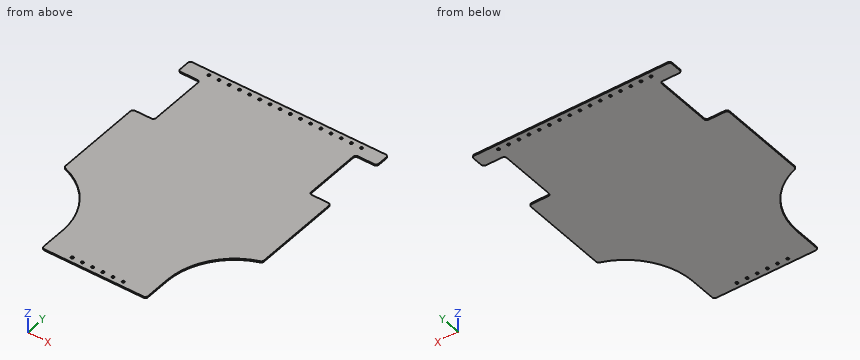
from build123d import *

# Parameters (mm, degrees)
BOSS_EXTRUDE1_DEPTH = 3.175
CUT_EXTRUDE1_DEPTH  = 403.674624387
SKETCH3_W           = 260.35
SKETCH3_H           = 3.175
BOSS_EXTRUDE2_DEPTH = 12.7
FILLET1_R           = 6.35
SKETCH5_R           = 3.175
CUT_EXTRUDE2_DEPTH  = 413.762211358


with BuildPart() as part:
    # Sketch1 → Boss-Extrude1 (new body)
    with BuildSketch(Plane.XY):
        Polygon((-247.65, 127), (-247.65, -317.5), (247.65, -317.5), (247.65, 127), (193.675, 127), (193.675, 279.4), (247.65, 279.4), (247.65, 317.5), (-247.65, 317.5), (-247.65, 279.4), (-193.675, 279.4), (-193.675, 127), align=None)
    extrude(amount=BOSS_EXTRUDE1_DEPTH)

    # Sketch2 → Cut-Extrude1 (cut, through all)
    with BuildSketch(Plane(origin=(0, 0, 0), x_dir=(-1, 0, 0), z_dir=(0, 0, -1))):
        with BuildLine():
            Line((-130.175, -260.35), (-130.175, -324.332629374))
            Line((-130.175, -324.332629374), (-142.81356865, -324.332629374))
            ThreePointArc((-142.81356865, -324.332629374), (-463.535123664, -227.740529446), (-130.175, -260.35))
        make_face()
        with BuildLine():
            Line((130.175, -324.332629374), (142.81356865, -324.332629374))
            ThreePointArc((142.81356865, -324.332629374), (463.535123664, -227.740529446), (130.175, -260.35))
            Line((130.175, -260.35), (130.175, -324.332629374))
        make_face()
    extrude(amount=-CUT_EXTRUDE1_DEPTH, mode=Mode.SUBTRACT)

    # Sketch3 → Boss-Extrude2 (add)
    with BuildSketch(Plane.XZ.offset(317.5)):
        with Locations((0, 1.5875)):
            Rectangle(SKETCH3_W, SKETCH3_H)
    extrude(amount=BOSS_EXTRUDE2_DEPTH)

    # Fillet1
    fillet1_edges = [part.edges().sort_by_distance(p)[0] for p in [
        (-247.65, 317.5, 1.5875),
        (247.65, 317.5, 1.5875),
        (247.65, 279.4, 1.5875),
        (193.675, 279.4, 1.5875),
        (193.675, 127, 1.5875),
        (247.65, 127, 1.5875),
        (-247.65, 127, 1.5875),
        (-193.675, 127, 1.5875),
        (-193.675, 279.4, 1.5875),
        (-247.65, 279.4, 1.5875),
        (247.65, -99.926075272, 1.5875),
        (-247.65, -99.926075272, 1.5875),
        (-130.175, -330.2, 1.5875),
        (130.175, -330.2, 1.5875),
    ]]
    fillet(fillet1_edges, radius=FILLET1_R)

    # Sketch5 → Cut-Extrude2 (cut, through all)
    with BuildSketch(Plane(origin=(0, 0, 0), x_dir=(-1, 0, 0), z_dir=(0, 0, -1))):
        with Locations((63.5, -317.5)):
            Circle(SKETCH5_R)
        with Locations((38.1, -317.5)):
            Circle(SKETCH5_R)
        with Locations((12.7, -317.5)):
            Circle(SKETCH5_R)
        with Locations((-12.7, -317.5)):
            Circle(SKETCH5_R)
        with Locations((-38.1, -317.5)):
            Circle(SKETCH5_R)
        with Locations((-63.5, -317.5)):
            Circle(SKETCH5_R)
        with Locations((190.5, 304.8)):
            Circle(SKETCH5_R)
        with Locations((165.1, 304.8)):
            Circle(SKETCH5_R)
        with Locations((139.7, 304.8)):
            Circle(SKETCH5_R)
        with Locations((114.3, 304.8)):
            Circle(SKETCH5_R)
        with Locations((88.9, 304.8)):
            Circle(SKETCH5_R)
        with Locations((63.5, 304.8)):
            Circle(SKETCH5_R)
        with Locations((38.1, 304.8)):
            Circle(SKETCH5_R)
        with Locations((12.7, 304.8)):
            Circle(SKETCH5_R)
        with Locations((-12.7, 304.8)):
            Circle(SKETCH5_R)
        with Locations((-38.1, 304.8)):
            Circle(SKETCH5_R)
        with Locations((-63.5, 304.8)):
            Circle(SKETCH5_R)
        with Locations((-88.9, 304.8)):
            Circle(SKETCH5_R)
        with Locations((-114.3, 304.8)):
            Circle(SKETCH5_R)
        with Locations((-139.7, 304.8)):
            Circle(SKETCH5_R)
        with Locations((-165.1, 304.8)):
            Circle(SKETCH5_R)
        with Locations((-190.5, 304.8)):
            Circle(SKETCH5_R)
    extrude(amount=-CUT_EXTRUDE2_DEPTH, mode=Mode.SUBTRACT)


solid = part.part
Geometry check sheet. Reference: the model listing, model coordinates, mm. Give positions to 0.01 mm unless a question says otherwise; leave off trailing zeros. Order: outer loops, then holes, each group sorted by start corner. A loop starts at its lowest first (then second) coordinate and runs counter-clockwise, first axis right, second up. Notation, with made-up numbers: M -11.5,39.25 L 20.5,39.25 A25 cw 20.5,51.25 Z; hole C 81,-7 d11. An arc over 180 degrees is marked long. Use a Markdown table: item, result.
Item 1: Section check A-A (y = 216.5). Record the cut outline in (x, z) (3 decimals), and give its area (3 significant figures).
Answers follow:
| item | result |
|---|---|
| outline | M -193.675,0 L 193.675,0 L 193.675,3.175 L -193.675,3.175 Z |
| area | 1,230 mm2 |
Item 2: Depth check by flat-ended pin: P1, Ø1, axis at y = -289.5, z = 2, coming from the -X side (3 decimals). Enter the tip coordinate at first touch or a pass-through.
Answers follow:
| item | result |
|---|---|
| P1 | stops at x = -130.175 |
Item 3: Material ranges on line 1 along Y through (x, z) = (63.5, 1.5) (3 decimals); line 2 along Y through (x, z) = (91, 2.2); line 3 along Y through (x, z) = (-198, 1.95), recorded low to high.
Answers follow:
| item | result |
|---|---|
| line 1 | y = -330.2 to -320.675, -314.325 to 301.625, 307.975 to 317.5 |
| line 2 | y = -330.2 to 302.42, 307.18 to 317.5 |
| line 3 | y = -125.35 to 127.33, 279.07 to 317.5 |
Item 4: Section check B-B (z = 1.8). State how many separate pieces and enclosed holes the cut face has, and give its area (3 significant figures).
Answers follow:
| item | result |
|---|---|
| separate pieces | 1 |
| enclosed holes | 22 |
| area | 260,000 mm2 |
